For this review, take the finished solid that the model builds, in its own axes (mm). Face numbers are marked on the shaded views. A direction names the side the tool comes from. Give positions to 0.01 mm unless a question says otherwise; leave off trailing zeros. Loops run counter-clockwise (first coordinate to the right, second up) from the corner with the lowest first, then second, coordinate; pieces in that order, holes last.
```python
from build123d import *

# Parameters (mm, degrees)
BASE_FLANGE1_DEPTH             = 57
EDGE_FLANGE1_STRIP_W           = 18
EDGE_FLANGE1_STRIP_H           = 3
EDGE_FLANGE1_STRIP_CUT_DEPTH   = 57
EDGE_FLANGE1_STRIP_2_W         = 18
EDGE_FLANGE1_STRIP_2_H         = 3
EDGE_FLANGE1_STRIP_CUT_2_DEPTH = 57
EDGE_FLANGE1_DEPTH             = 57
EDGE_FLANGE1_BEND_DEPTH        = 57
CUT_EXTRUDE1_REACH             = 93.328
SKETCH12_R                     = 10
CHAMFER1_SIZE                  = 30
CUT_EXTRUDE2_REACH             = 92.922
SKETCH13_R                     = 5
FILLET1_R                      = 3


# Sheet-metal steps are written as plain solids
with BuildPart() as part:
    # Sketch1 → Base-Flange1 (new body)
    with BuildSketch(Plane(origin=(0, 0, 0), x_dir=(1, 0, 0), z_dir=(0, 1, 0))):
        with BuildLine():
            Line((-20, 0), (-20, 7.85))
            ThreePointArc((-20, 7.85), (-19.121320344, 9.971320344), (-17, 10.85))
            Line((-17, 10.85), (17, 10.85))
            ThreePointArc((17, 10.85), (19.121320344, 9.971320344), (20, 7.85))
            Line((20, 7.85), (20, 0))
            Line((20, 0), (23, 0))
            Line((23, 0), (23, 7.85))
            ThreePointArc((23, 7.85), (21.242640687, 12.092640687), (17, 13.85))
            Line((17, 13.85), (-17, 13.85))
            ThreePointArc((-17, 13.85), (-21.242640687, 12.092640687), (-23, 7.85))
            Line((-23, 7.85), (-23, 0))
            Line((-23, 0), (-20, 0))
        make_face()
    extrude(amount=BASE_FLANGE1_DEPTH)

    # Edge-Flange1 strip (across the edge) → Edge-Flange1 strip cut (cut)
    with BuildSketch(Plane(origin=(23, 57, 0), x_dir=(0, 0, -1), z_dir=(0, -1, 0))):
        with Locations((-3, -1.5)):
            Rectangle(EDGE_FLANGE1_STRIP_W, EDGE_FLANGE1_STRIP_H)
    extrude(amount=EDGE_FLANGE1_STRIP_CUT_DEPTH, mode=Mode.SUBTRACT)

    # Edge-Flange1 strip 2 (across the edge) → Edge-Flange1 strip cut 2 (cut)
    with BuildSketch(Plane(origin=(-23, 0, 0), x_dir=(0, 0, -1), z_dir=(0, 1, 0))):
        with Locations((-3, -1.5)):
            Rectangle(EDGE_FLANGE1_STRIP_2_W, EDGE_FLANGE1_STRIP_2_H)
    extrude(amount=EDGE_FLANGE1_STRIP_CUT_2_DEPTH, mode=Mode.SUBTRACT)

    # Edge-Flange1 section (across the edge) → Edge-Flange1 (add)
    with BuildSketch(Plane(origin=(23, 57, 0), x_dir=(0, 0, -1), z_dir=(0, -1, 0))):
        with BuildLine():
            Line((0, 3), (0, 47))
            Line((0, 47), (3, 47))
            Line((3, 47), (3, 3))
            ThreePointArc((3, 3), (3.878679656, 0.878679656), (6, 0))
            Line((6, 0), (6, -3))
            ThreePointArc((6, -3), (1.757359313, -1.242640687), (0, 3))
        make_face()
    extrude(amount=EDGE_FLANGE1_DEPTH)

    # Edge-Flange1 section 2 (across the edge) → Edge-Flange1 bend (add)
    with BuildSketch(Plane(origin=(-23, 0, 0), x_dir=(0, 0, -1), z_dir=(0, 1, 0))):
        with BuildLine():
            Line((0, 3), (0, 47))
            Line((0, 47), (3, 47))
            Line((3, 47), (3, 3))
            ThreePointArc((3, 3), (3.878679656, 0.878679656), (6, 0))
            Line((6, 0), (6, -3))
            ThreePointArc((6, -3), (1.757359313, -1.242640687), (0, 3))
        make_face()
    extrude(amount=EDGE_FLANGE1_BEND_DEPTH)

    # Sketch12 → Cut-Extrude1 (cut, up to next)
    with BuildSketch(Plane(origin=(0, 0, -13.85), x_dir=(-1, 0, 0), z_dir=(0, 0, -1)), mode=Mode.PRIVATE) as cut_extrude1_sk1:
        with Locations((0, 37)):
            Circle(SKETCH12_R)
    cut_extrude1_tool1 = extrude(cut_extrude1_sk1.sketch, amount=-CUT_EXTRUDE1_REACH, mode=Mode.PRIVATE) & part.part
    add(cut_extrude1_tool1.solids().sort_by_distance((0, 37, -13.85))[0], mode=Mode.SUBTRACT)

    # Chamfer1
    chamfer1_edges = [part.edges().sort_by_distance(p)[0] for p in [
        (70, 57, -1.5),
        (-70, 57, -1.5),
    ]]
    chamfer(chamfer1_edges, length=CHAMFER1_SIZE)

    # Sketch13 → Cut-Extrude2 (cut, up to next)
    with BuildSketch(Plane(origin=(0, 0, -3), x_dir=(-1, 0, 0), z_dir=(0, 0, -1)), mode=Mode.PRIVATE) as cut_extrude2_sk1:
        with Locations((-61, 16)):
            Circle(SKETCH13_R)
    cut_extrude2_tool1 = extrude(cut_extrude2_sk1.sketch, amount=-CUT_EXTRUDE2_REACH, mode=Mode.PRIVATE) & part.part
    # Sketch13 → Cut-Extrude2 (cut, up to next)
    with BuildSketch(Plane(origin=(0, 0, -3), x_dir=(-1, 0, 0), z_dir=(0, 0, -1)), mode=Mode.PRIVATE) as cut_extrude2_sk2:
        with Locations((-41, 16)):
            Circle(SKETCH13_R)
    cut_extrude2_tool2 = extrude(cut_extrude2_sk2.sketch, amount=-CUT_EXTRUDE2_REACH, mode=Mode.PRIVATE) & part.part
    # Sketch13 → Cut-Extrude2 (cut, up to next)
    with BuildSketch(Plane(origin=(0, 0, -3), x_dir=(-1, 0, 0), z_dir=(0, 0, -1)), mode=Mode.PRIVATE) as cut_extrude2_sk3:
        with Locations((41, 16)):
            Circle(SKETCH13_R)
    cut_extrude2_tool3 = extrude(cut_extrude2_sk3.sketch, amount=-CUT_EXTRUDE2_REACH, mode=Mode.PRIVATE) & part.part
    # Sketch13 → Cut-Extrude2 (cut, up to next)
    with BuildSketch(Plane(origin=(0, 0, -3), x_dir=(-1, 0, 0), z_dir=(0, 0, -1)), mode=Mode.PRIVATE) as cut_extrude2_sk4:
        with Locations((61, 16)):
            Circle(SKETCH13_R)
    cut_extrude2_tool4 = extrude(cut_extrude2_sk4.sketch, amount=-CUT_EXTRUDE2_REACH, mode=Mode.PRIVATE) & part.part
    add(cut_extrude2_tool1.solids().sort_by_distance((61, 16, -3))[0], mode=Mode.SUBTRACT)
    add(cut_extrude2_tool2.solids().sort_by_distance((41, 16, -3))[0], mode=Mode.SUBTRACT)
    add(cut_extrude2_tool3.solids().sort_by_distance((-41, 16, -3))[0], mode=Mode.SUBTRACT)
    add(cut_extrude2_tool4.solids().sort_by_distance((-61, 16, -3))[0], mode=Mode.SUBTRACT)

    # Fillet1
    fillet1_edges = [part.edges().sort_by_distance(p)[0] for p in [
        (-70, 27, -1.5),
        (-40, 57, -1.5),
        (40, 57, -1.5),
        (70, 27, -1.5),
        (70, 0, -1.5),
        (-70, 0, -1.5),
    ]]
    fillet(fillet1_edges, radius=FILLET1_R)


solid = part.part
```
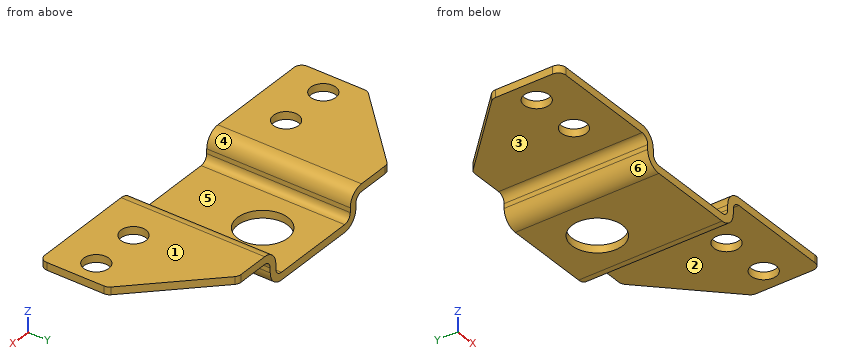
Q1. For pin 1 Ø17 at (x, y) = (6, 14.5) entering from +Z; pin 2 Ø4 at (x, y) = (-49.5, 17.5) entering from -Z; pin 3 Ø0.9 at (y, z) = (24, -6.5) entering from -X, all flat-tipped, find the tip position at first contact; note any pin that passes through.
Answers:
pin 1: stops at z = -10.85
pin 2: stops at z = -3
pin 3: stops at x = -23
Q2. Consider section B-B on x = 61. Give the boundary of the cut face in (y, z).
Answers:
outline: (0, -3) - (11, -3) - (11, 0) - (0, 0) - close; (21, -3) - (36, -3) - (36, 0) - (21, 0) - close
Q3. Consider section A-A on y = 37. Give the boundary of the cut face in (x, z).
Answers:
outline: (-60, -3) - (-26, -3) arc R3 cw to (-23, -6) - (-23, -7.85) arc R6 ccw to (-17, -13.85) - (-10, -13.85) - (-10, -10.85) - (-17, -10.85) arc R3 cw to (-20, -7.85) - (-20, -6) arc R6 ccw to (-26, 0) - (-60, 0) - close; (10, -13.85) - (17, -13.85) arc R6 ccw to (23, -7.85) - (23, -6) arc R3 cw to (26, -3) - (60, -3) - (60, 0) - (26, 0) arc R6 ccw to (20, -6) - (20, -7.85) arc R3 cw to (17, -10.85) - (10, -10.85) - close
Q4. Machinability: for the marked faces 1 and 2, which of the approach directions +Z, -Z, +X, -X, +Y, -Y give a long, thin tool a straight path to every point of the face, cutting with its end or side? Answer none if there is none.
Answers:
face 1: +Z, +X, -X, +Y, -Y
face 2: -Z, +X, +Y, -Y
Q5. For probe 1 along X at (y, z) = (23, -7.5); probe 2 along Y at (x, z) = (41, -1.85); probe 3 along Y at (x, z) = (-61, -1.4), list the stretches that pass through material, from the lowest coordinate up.
Answers:
probe 1: x = -23 to -20, 20 to 23
probe 2: y = 0 to 11, 21 to 56
probe 3: y = 0 to 11, 21 to 36
Q6. Consider section D-D on x = 0. Give the boundary of the cut face in (y, z).
Answers:
outline: (0, -13.85) - (27, -13.85) - (27, -10.85) - (0, -10.85) - close; (47, -13.85) - (57, -13.85) - (57, -10.85) - (47, -10.85) - close
Q7. Mouldability with a two-part tool opening along X and no side actions: class the marked faces 3, 4, 5 and 6 as +X half, -X half, draft (parallel to the pull), parting line (faces both ways), or undercut.
Answers:
face 3: draft
face 4: undercut
face 5: undercut
face 6: -X half
Q8. Consider section C-C on y = 45. Give the boundary of the cut face in (x, z).
Answers:
outline: (-52, -3) - (-26, -3) arc R3 cw to (-23, -6) - (-23, -7.85) arc R6 ccw to (-17, -13.85) - (-6, -13.85) - (-6, -10.85) - (-17, -10.85) arc R3 cw to (-20, -7.85) - (-20, -6) arc R6 ccw to (-26, 0) - (-52, 0) - close; (6, -13.85) - (17, -13.85) arc R6 ccw to (23, -7.85) - (23, -6) arc R3 cw to (26, -3) - (52, -3) - (52, 0) - (26, 0) arc R6 ccw to (20, -6) - (20, -7.85) arc R3 cw to (17, -10.85) - (6, -10.85) - close
